from build123d import *

# Parameters (mm, degrees)
F0_W     = 60
F0_H     = 20
F0_R     = 2.6
F1_DEPTH = 6
F2_R     = 4.5
F3_DEPTH = 2
F5_DEPTH = 60.001


with BuildPart() as f1:
    # F0 (on Right) → F1 (new body)
    with BuildSketch(Plane.YZ):
        Rectangle(F0_W, F0_H)
        with Locations((-20, 0)):
            Circle(F0_R, mode=Mode.SUBTRACT)
        Circle(F0_R, mode=Mode.SUBTRACT)
        with Locations((20, 0)):
            Circle(F0_R, mode=Mode.SUBTRACT)
    extrude(amount=F1_DEPTH)

    # F2 (on face) → F3 (cut)
    with BuildSketch(Plane.YZ.offset(6)):
        with Locations((-20, 0)):
            Circle(F2_R)
        Circle(F2_R)
        with Locations((20, 0)):
            Circle(F2_R)
    extrude(amount=-F3_DEPTH, mode=Mode.SUBTRACT)

    # F4 (on face) → F5 (cut, through all)
    with BuildSketch(Plane.XZ.offset(30)):
        Polygon((6, 8.5), (4.5, 7), (6, 5.5), align=None)
        Polygon((6, -8.5), (6, -5.5), (4.5, -7), align=None)
    extrude(amount=-F5_DEPTH, mode=Mode.SUBTRACT)


solid = f1.part
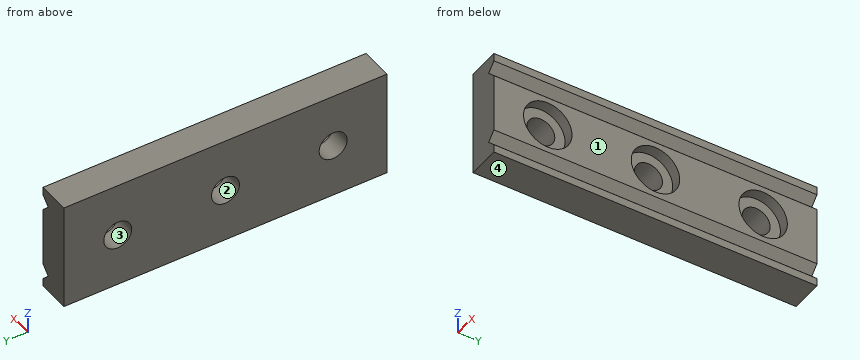
CAD build for the part. Positions are in the model's coordinates, mm. Face numbers are marked on the shaded views. Give positions to 0.01 mm unless a question says otherwise; leave off trailing zeros. Loops run counter-clockwise (first coordinate to the right, second up) from the corner with the lowest first, then second, coordinate; pieces in that order, holes last. Notation, with made-up numbers: M -25,60.25 L 1,60.25 A23 ccw 1,84.25 Z; hole C 68,31 d10. An arc over 180 degrees is marked long. Answer in a Markdown table with one row per item. Add a question column.
Item 1: Band-saw the part on D-D on y = 10. Give the cut face in (x, z).
Item 2: Drop flat-ended pins along their axis: P1, Ø1.5, axis at y = 4, z = 0, coming from the -X side; P2, Ø4, axis at y = 0, z = 0, coming from the +X side; P3, Ø2.5, axis at y = -1, z = 1.5, coming from the +X side. Give the stop position or say it passes through.
Item 3: Band-saw the part on B-B on y = 0. Give the cut face in (x, z).
Item 4: Band-saw the part on C-C on x = 1.9. Give the cut face in (y, z).
Item 5: Probe probe 1 along Y at (x, z) = (1.5, 0); probe 2 along Z at (x, y) = (2.8, 20); probe 3 along Z at (x, y) = (5.05, -20). List the from-to ranges inside material, lowest first.
Item 6: Mould opens along Z. For the marked faces 1, 2, 3 and 4 say: +Z half, -Z half, draft (parallel to the pull), parting line (faces both ways), or undercut.
Item 7: Band-saw the part on A-A on z = 0. Give the cut face in (x, y), then the cut area to 3 significant figures.
Reply:
| question | item | result |
|---|---|---|
| 1 | outline | M 0,-10 L 6,-10 L 6,-8.5 L 4.5,-7 L 6,-5.5 L 6,5.5 L 4.5,7 L 6,8.5 L 6,10 L 0,10 Z |
| 2 | P1 | stops at x = 0 |
| 2 | P2 | passes through |
| 2 | P3 | stops at x = 4 |
| 3 | outline | M 0,-10 L 6,-10 L 6,-8.5 L 4.5,-7 L 6,-5.5 L 6,-4.5 L 4,-4.5 L 4,-2.6 L 0,-2.6 Z; M 0,2.6 L 4,2.6 L 4,4.5 L 6,4.5 L 6,5.5 L 4.5,7 L 6,8.5 L 6,10 L 0,10 Z |
| 4 | outline | M -30,-10 L 30,-10 L 30,10 L -30,10 Z; hole C -20,0 d5.2; hole C 0,0 d5.2; hole C 20,0 d5.2 |
| 5 | probe 1 | y = -30 to -22.6, -17.4 to -2.6, 2.6 to 17.4, 22.6 to 30 |
| 5 | probe 2 | z = -10 to -2.6, 2.6 to 10 |
| 5 | probe 3 | z = -10 to -7.55, -6.45 to -4.5, 4.5 to 6.45, 7.55 to 10 |
| 6 | face 1 | draft |
| 6 | face 2 | undercut |
| 6 | face 3 | undercut |
| 6 | face 4 | -Z half |
| 7 | outline | M 0,-30 L 6,-30 L 6,-24.5 L 4,-24.5 L 4,-22.6 L 0,-22.6 Z; M 0,-17.4 L 4,-17.4 L 4,-15.5 L 6,-15.5 L 6,-4.5 L 4,-4.5 L 4,-2.6 L 0,-2.6 Z; M 0,2.6 L 4,2.6 L 4,4.5 L 6,4.5 L 6,15.5 L 4,15.5 L 4,17.4 L 0,17.4 Z; M 0,22.6 L 4,22.6 L 4,24.5 L 6,24.5 L 6,30 L 0,30 Z |
| 7 | area | 244 mm^2 |
